Work out the finished part from the listing and answer in its coordinate system (mm). Face numbers are marked on the shaded views. A direction names the side the tool comes from. Coordinates: 2 decimals unless noted, no trailing zeros. Order: outer loops, then holes, each group sorted by start corner. A loop starts at its lowest first (then second) coordinate and runs counter-clockwise, first axis right, second up.
1. Flat-ended cylindrical pins translate along their axes: pin 1 Ø8 at (x, y) = (-16, 9) entering from +Z; pin 2 Ø4.5 at (x, z) = (-1.5, 37) entering from +Y; pin 3 Ø6 at (y, z) = (-3, 32) entering from +X. Find the tip coordinate at first contact, or state that the pin passes through.
2. The part is cut by section D-D, the plane y = 4. Give the vertices of the cut face in (x, z).
3. The part is cut by section B-B, the plane x = 27.5. Give the vertices of the cut face in (y, z).
4. Find the intervals of material crossed by probe 1 along Z at (x, y) = (11, -7); probe 2 along X at (y, z) = (-4, 17); probe 3 along X at (y, z) = (-4.5, 47.5), in increasing order.
5. A tool of negligible diameter and unlimited length cuts with its end or side. For the marked faces 1 and 2, from which of +Z, -Z, +X, -X, +Y, -Y can it reach the whole face along a straight path? Write none if from no direction.
6. The part is cut by section C-C, the plane z = 12. Give the vertices of the cut face in (x, y), then the cut area to 3 significant figures.
7. The part is cut by section A-A, the plane y = -2. Give the vertices of the cut face in (x, z).
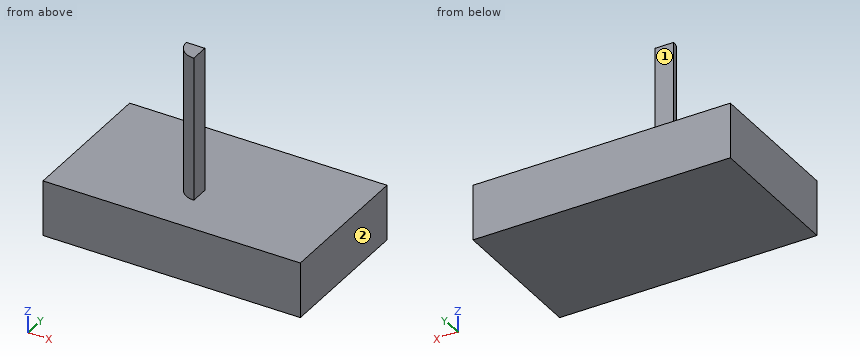
```python
from build123d import *

# Parameters (mm, degrees)
F1_DEPTH      = 16.98069
F1_DEPTH_BACK = 25.4
F2_W          = 5.4000006057
F2_H          = 50.1300022006
F3_ANGLE      = 90


with BuildPart() as f1:
    # F0 (on Front) → F1 (new body, two sides)
    with BuildSketch(Plane.XZ) as f1_sk:
        Polygon((-37.080001086, -8.1900004297), (37.9800014198, -8.1900004297), (37.9800014198, 8.0099999905), (0, 8.0099999905), (-37.080001086, 8.0099999905), align=None)
    extrude(amount=F1_DEPTH)
    extrude(f1_sk.sketch, amount=-F1_DEPTH_BACK)

    # F2 (on Front) → F3 (revolve)
    with BuildSketch(Plane.XZ):
        with Locations((-2.7000003029, 25.0650011003)):
            Rectangle(F2_W, F2_H)
    revolve(axis=Axis((0, 0, 25.0650011003), (0, 0, 1)), revolution_arc=F3_ANGLE)


solid = f1.part
```
Geometry says:
1. pin 1: stops at z = 8.01
1. pin 2: stops at y = 0
1. pin 3: stops at x = 0
2. outline: (-37.08, -8.19) - (37.98, -8.19) - (37.98, 8.01) - (-37.08, 8.01) - close
3. outline: (-16.98, -8.19) - (25.4, -8.19) - (25.4, 8.01) - (-16.98, 8.01) - close
4. probe 1: z = -8.19 to 8.01
4. probe 2: x = -3.63 to 0
4. probe 3: x = -2.98 to 0
5. face 1: +Z, +X, -X, +Y
5. face 2: +Z, -Z, +X, +Y, -Y
6. outline: (-5.4, 0) arc R5.4 ccw to (0, -5.4) - (0, 0) - close
6. area: 22.9 mm2
7. outline: (-37.08, -8.19) - (37.98, -8.19) - (37.98, 8.01) - (0, 8.01) - (0, 50.13) - (-5.02, 50.13) - (-5.02, 8.01) - (-37.08, 8.01) - close
